The listing builds one solid part. Answer for the finished solid, in the listing's coordinates (mm). Face numbers are marked on the shaded views. Round coordinates to 2 decimals unless told otherwise and drop trailing zeros.
(1) A cutting plane is placed at A-A, the plane y = 14. Give the number of separate pieces and of enclosed holes in the cut face, and give its area (3 significant figures).
(2) Each of these flat-tipped pins is pushed along its axis until it touches: pin 1 Ø8 at (x, z) = (-48.01, -44.53) entering from +Y (3 decimals); pin 2 Ø3 at (x, z) = (-46, -40.5) entering from -Y (3 decimals); pin 3 Ø8.5 at (x, z) = (60.71, -57.23) entering from -Y. Where does it stop, or does it pass through?
(3) The mould has two halves that part along Z. Classify the marked faces 1, 2, 3 and 4: +Z half, -Z half, draft (parallel to the pull), parting line (faces both ways), or undercut.
(4) Find the intervals of material crossed by probe 1 along X at (y, z) = (12.5, -33.5); probe 2 along Z at (x, y) = (23, 18.5); probe 3 along Z at (x, y) = (-25.4, 12.5), in increasing order.
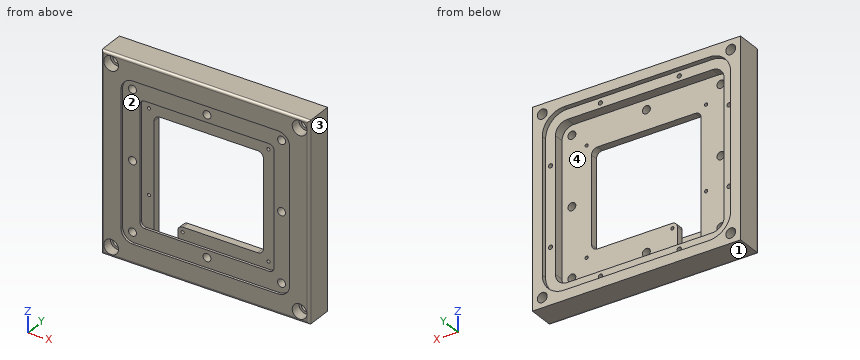
from build123d import *

# Parameters (mm, degrees)
SKETCH2_W                                            = 134.112
SKETCH2_H                                            = 127.1524
SKETCH2_W_2                                          = 83.312
SKETCH2_H_2                                          = 76.3524
SKETCH2_W_3                                          = 21.7424
SKETCH2_H_3                                          = 15.9766
BOSS_EXTRUDE1_DEPTH                                  = 15.875
BOSS_EXTRUDE2_DEPTH                                  = 9.525
CUT_EXTRUDE2_DEPTH                                   = 3.175
M2_5X0_45_TAPPED_HOLE1_D                             = 2.05
M2_5X0_45_TAPPED_HOLE1_DEPTH                         = 6.35
M2_5X0_45_TAPPED_HOLE1_TIP                           = 0.615882135
F_10_CLEARANCE_HOLE1_D                               = 5.1054
CUT_EXTRUDE3_DEPTH                                   = 6.35
CUT_EXTRUDE4_DEPTH                                   = 1.6
SKETCH12_W                                           = 70.612
SKETCH12_H                                           = 63.6524
CUT_EXTRUDE5_DEPTH                                   = 12.1
FILLET1_R                                            = 3.81
SKETCH13_W                                           = 134.112
SKETCH13_H                                           = 127.1524
CUT_EXTRUDE6_DEPTH                                   = 1.5875
FILLET2_R                                            = 1.5875
SKETCH14_W                                           = 15.3924
SKETCH14_H                                           = 22.86
CUT_EXTRUDE7_DEPTH                                   = 4.75
FILLET3_R                                            = 3.175
SKETCH15_W                                           = 134.112
SKETCH15_H                                           = 127.1524
BOSS_EXTRUDE3_DEPTH                                  = 3.175
F_6_32_TAPPED_HOLE1_AT_2_COUNT                       = 2
F_6_32_TAPPED_HOLE1_AT_2_PITCH                       = 108.1024
F_6_32_TAPPED_HOLE1_AT_3_COUNT                       = 2
F_6_32_TAPPED_HOLE1_AT_3_PITCH                       = 85.702359025
F_6_32_TAPPED_HOLE1_AT_4_COUNT                       = 2
F_6_32_TAPPED_HOLE1_AT_4_PITCH                       = 43.049882955
CBORE_FOR_1_4_BINDING_HEAD_MACHINE_SCREW_D           = 6.35
CBORE_FOR_1_4_BINDING_HEAD_MACHINE_SCREW_DEPTH       = 17.4625
CBORE_FOR_1_4_BINDING_HEAD_MACHINE_SCREW_CBORE_D     = 9.525
CBORE_FOR_1_4_BINDING_HEAD_MACHINE_SCREW_CBORE_DEPTH = 6.35


with BuildPart() as part:
    # Sketch2 → Boss-Extrude1 (new body)
    with BuildSketch(Plane(origin=(0, 0, 0), x_dir=(1, 0, 0), z_dir=(0, 1, 0))):
        Rectangle(SKETCH2_W, SKETCH2_H)
        Rectangle(SKETCH2_W_2, SKETCH2_H_2, mode=Mode.SUBTRACT)
        with Locations((-30.7848, 30.1879)):
            Rectangle(SKETCH2_W_3, SKETCH2_H_3)
    extrude(amount=BOSS_EXTRUDE1_DEPTH)

    # Sketch4 → Boss-Extrude2 (add)
    with BuildSketch(Plane(origin=(0, 0, 0), x_dir=(1, 0, 0), z_dir=(0, 1, 0))):
        Polygon((41.656, -38.1762), (41.656, 38.1762), (-19.9136, 38.1762), (-19.9136, 22.1996), (-41.656, 22.1996), (-41.656, -38.1762), align=None)
        Polygon((35.306, 31.8262), (-13.5636, 31.8262), (-13.5636, 15.8496), (-35.306, 15.8496), (-35.306, -31.8262), (35.306, -31.8262), align=None, mode=Mode.SUBTRACT)
    extrude(amount=BOSS_EXTRUDE2_DEPTH)

    # Sketch5 → Cut-Extrude2 (cut)
    with BuildSketch(Plane.XZ):
        with BuildLine():
            Line((46.736, -50.8762), (-46.736, -50.8762))
            ThreePointArc((-46.736, -50.8762), (-52.124153673, -48.644353673), (-54.356, -43.2562))
            Line((-54.356, -43.2562), (-54.356, 43.2562))
            ThreePointArc((-54.356, 43.2562), (-52.124153673, 48.644353673), (-46.736, 50.8762))
            Line((-46.736, 50.8762), (46.736, 50.8762))
            ThreePointArc((46.736, 50.8762), (52.124153673, 48.644353673), (54.356, 43.2562))
            Line((54.356, 43.2562), (54.356, -43.2562))
            ThreePointArc((54.356, -43.2562), (52.124153673, -48.644353673), (46.736, -50.8762))
        make_face()
    extrude(amount=-CUT_EXTRUDE2_DEPTH, mode=Mode.SUBTRACT)

    # M2.5x0.45 Tapped Hole1
    with Locations(Plane(origin=(0, 3.175, 0), x_dir=(-1, 0, 0), z_dir=(0, -1, 0))):
        with Locations((38.481, -35.0012), (-38.481, -35.0012), (38.481, 19.0246), (16.7386, 35.0012), (-38.481, 35.0012)):
            Hole(M2_5X0_45_TAPPED_HOLE1_D / 2, depth=M2_5X0_45_TAPPED_HOLE1_DEPTH)
            with Locations((0, 0, -(M2_5X0_45_TAPPED_HOLE1_DEPTH + M2_5X0_45_TAPPED_HOLE1_TIP / 2))):  # 118° drill point
                Cone(0, M2_5X0_45_TAPPED_HOLE1_D / 2, M2_5X0_45_TAPPED_HOLE1_TIP, mode=Mode.SUBTRACT)

    # 10 Clearance Hole1 (through all)
    with Locations(Plane(origin=(0, 3.175, 0), x_dir=(-1, 0, 0), z_dir=(0, -1, 0))):
        with Locations((48.006, -44.5262), (0, -44.5262), (-48.006, -44.5262), (-48.006, 0), (-48.006, 44.5262), (0, 44.5262), (48.006, 44.5262), (48.006, 0)):
            Hole(F_10_CLEARANCE_HOLE1_D / 2)

    # Sketch10 → Cut-Extrude3 (cut)
    with BuildSketch(Plane(origin=(0, 15.875, 0), x_dir=(1, 0, 0), z_dir=(0, 1, 0))):
        with BuildLine():
            Line((54.356, -43.2562), (54.356, 43.2562))
            ThreePointArc((54.356, 43.2562), (52.124153673, 48.644353673), (46.736, 50.8762))
            Line((46.736, 50.8762), (-46.736, 50.8762))
            ThreePointArc((-46.736, 50.8762), (-52.124153673, 48.644353673), (-54.356, 43.2562))
            Line((-54.356, 43.2562), (-54.356, -43.2562))
            ThreePointArc((-54.356, -43.2562), (-52.124153673, -48.644353673), (-46.736, -50.8762))
            Line((-46.736, -50.8762), (46.736, -50.8762))
            ThreePointArc((46.736, -50.8762), (52.124153673, -48.644353673), (54.356, -43.2562))
        make_face()
    extrude(amount=-CUT_EXTRUDE3_DEPTH, mode=Mode.SUBTRACT)

    # Sketch11 → Cut-Extrude4 (cut)
    with BuildSketch(Plane.XZ.offset(-3.175)):
        with BuildLine():
            Line((40.0685, 39.7637), (-40.0685, 39.7637))
            ThreePointArc((-40.0685, 39.7637), (-42.31356403, 38.83376403), (-43.2435, 36.5887))
            Line((-43.2435, 36.5887), (-43.2435, -36.5887))
            ThreePointArc((-43.2435, -36.5887), (-42.31356403, -38.83376403), (-40.0685, -39.7637))
            Line((-40.0685, -39.7637), (40.0685, -39.7637))
            ThreePointArc((40.0685, -39.7637), (42.31356403, -38.83376403), (43.2435, -36.5887))
            Line((43.2435, -36.5887), (43.2435, 36.5887))
            ThreePointArc((43.2435, 36.5887), (42.31356403, 38.83376403), (40.0685, 39.7637))
        make_face()
    extrude(amount=-CUT_EXTRUDE4_DEPTH, mode=Mode.SUBTRACT)

    # Sketch12 → Cut-Extrude5 (cut, through all)
    with BuildSketch(Plane.XZ.offset(-4.775)):
        Rectangle(SKETCH12_W, SKETCH12_H)
    extrude(amount=-CUT_EXTRUDE5_DEPTH, mode=Mode.SUBTRACT)

    # Fillet1
    fillet1_edges = [part.edges().sort_by_distance(p)[0] for p in [
        (-35.306, 7.15, -31.8262),
        (35.306, 7.15, -31.8262),
        (-35.306, 7.15, 31.8262),
        (35.306, 7.15, 31.8262),
    ]]
    fillet(fillet1_edges, radius=FILLET1_R)

    # Sketch13 → Cut-Extrude6 (cut)
    with BuildSketch(Plane.XZ):
        Rectangle(SKETCH13_W, SKETCH13_H)
        with BuildLine():
            Line((54.356, -43.2562), (54.356, 43.2562))
            ThreePointArc((54.356, 43.2562), (52.124153673, 48.644353673), (46.736, 50.8762))
            Line((46.736, 50.8762), (-46.736, 50.8762))
            ThreePointArc((-46.736, 50.8762), (-52.124153673, 48.644353673), (-54.356, 43.2562))
            Line((-54.356, 43.2562), (-54.356, -43.2562))
            ThreePointArc((-54.356, -43.2562), (-52.124153673, -48.644353673), (-46.736, -50.8762))
            Line((-46.736, -50.8762), (46.736, -50.8762))
            ThreePointArc((46.736, -50.8762), (52.124153673, -48.644353673), (54.356, -43.2562))
        make_face(mode=Mode.SUBTRACT)
    extrude(amount=-CUT_EXTRUDE6_DEPTH, mode=Mode.SUBTRACT)

    # Fillet2
    fillet2_edges = [part.edges().sort_by_distance(p)[0] for p in [
        (67.056, 1.5875, 0),
        (0, 1.5875, -63.5762),
        (-67.056, 1.5875, 0),
        (0, 1.5875, 63.5762),
    ]]
    fillet(fillet2_edges, radius=FILLET2_R)

    # Sketch14 → Cut-Extrude7 (cut)
    with BuildSketch(Plane(origin=(0, 9.525, 0), x_dir=(1, 0, 0), z_dir=(0, 1, 0))):
        with Locations((-27.6098, 39.4462)):
            Rectangle(SKETCH14_W, SKETCH14_H)
    extrude(amount=-CUT_EXTRUDE7_DEPTH, mode=Mode.SUBTRACT)

    # Fillet3
    fillet3_edges = [part.edges().sort_by_distance(p)[0] for p in [
        (-19.9136, 7.15, -31.8262),
        (-19.9136, 7.15, -50.8762),
        (-35.306, 7.15, -50.8762),
    ]]
    fillet(fillet3_edges, radius=FILLET3_R)

    # Sketch15 → Boss-Extrude3 (add)
    with BuildSketch(Plane(origin=(0, 15.875, 0), x_dir=(1, 0, 0), z_dir=(0, 1, 0))):
        Rectangle(SKETCH15_W, SKETCH15_H)
        with BuildLine():
            ThreePointArc((46.736, -57.2262), (56.614281733, -53.134481733), (60.706, -43.2562))
            Line((60.706, -43.2562), (60.706, 43.2562))
            ThreePointArc((60.706, 43.2562), (56.614281733, 53.134481733), (46.736, 57.2262))
            Line((46.736, 57.2262), (-46.736, 57.2262))
            ThreePointArc((-46.736, 57.2262), (-56.614281733, 53.134481733), (-60.706, 43.2562))
            Line((-60.706, 43.2562), (-60.706, -43.2562))
            ThreePointArc((-60.706, -43.2562), (-56.614281733, -53.134481733), (-46.736, -57.2262))
            Line((-46.736, -57.2262), (46.736, -57.2262))
        make_face(mode=Mode.SUBTRACT)
    extrude(amount=BOSS_EXTRUDE3_DEPTH)

    # Sketch18 → 6-32 Tapped Hole1 (revolve, cut)
    with BuildSketch(Plane(origin=(-25.4, 15.875, 54.0512), x_dir=(0, 0, 1), z_dir=(1, 0, 0))):
        Polygon((0, 0), (0, 10.33769403), (1.35255, 9.525), (1.35255, 0), align=None)
    f_6_32_tapped_hole1 = revolve(axis=Axis((-25.4, 22.225, 54.0512), (0, -1, 0)), mode=Mode.SUBTRACT)

    # 6-32 Tapped Hole1 at 2: 6-32 Tapped Hole1 ×2
    with Locations(*[(0, 0, -i * F_6_32_TAPPED_HOLE1_AT_2_PITCH) for i in range(1, F_6_32_TAPPED_HOLE1_AT_2_COUNT)]):
        add(f_6_32_tapped_hole1, mode=Mode.SUBTRACT)

    # 6-32 Tapped Hole1 at 3: 6-32 Tapped Hole1 ×2
    with Locations(*[Vector(-0.374913834, 0, -0.927059662) * (i * F_6_32_TAPPED_HOLE1_AT_3_PITCH) for i in range(1, F_6_32_TAPPED_HOLE1_AT_3_COUNT)]):
        add(f_6_32_tapped_hole1, mode=Mode.SUBTRACT)

    # 6-32 Tapped Hole1 at 4: 6-32 Tapped Hole1 ×2
    with Locations(*[Vector(-0.746366721, 0, -0.665534911) * (i * F_6_32_TAPPED_HOLE1_AT_4_PITCH) for i in range(1, F_6_32_TAPPED_HOLE1_AT_4_COUNT)]):
        add(f_6_32_tapped_hole1, mode=Mode.SUBTRACT)

    # Mirror1: 6-32 Tapped Hole1 across plane
    add(f_6_32_tapped_hole1.mirror(Plane(origin=(0, 0, 0), x_dir=(0, 0, 1), z_dir=(1, 0, 0))), mode=Mode.SUBTRACT)

    # Mirror1 copy 1 sketch → Mirror1 copy 1 (revolve, cut)
    with BuildSketch(Plane(origin=(25.4, 15.875, -54.0512), x_dir=(0, 0, 1), z_dir=(-1, 0, 0))):
        Polygon((0, 0), (0, -10.33769403), (1.35255, -9.525), (1.35255, 0), align=None)
    revolve(axis=Axis((25.4, 22.225, -54.0512), (0, 1, 0)), mode=Mode.SUBTRACT)

    # Mirror1 copy 2 sketch → Mirror1 copy 2 (revolve, cut)
    with BuildSketch(Plane(origin=(57.531, 15.875, -25.4), x_dir=(0, 0, 1), z_dir=(-1, 0, 0))):
        Polygon((0, 0), (0, -10.33769403), (1.35255, -9.525), (1.35255, 0), align=None)
    revolve(axis=Axis((57.531, 22.225, -25.4), (0, 1, 0)), mode=Mode.SUBTRACT)

    # Mirror1 copy 3 sketch → Mirror1 copy 3 (revolve, cut)
    with BuildSketch(Plane(origin=(57.531, 15.875, 25.4), x_dir=(0, 0, 1), z_dir=(-1, 0, 0))):
        Polygon((0, 0), (0, -10.33769403), (1.35255, -9.525), (1.35255, 0), align=None)
    revolve(axis=Axis((57.531, 22.225, 25.4), (0, 1, 0)), mode=Mode.SUBTRACT)

    # CBORE for 1_4 Binding Head Machine Screw
    with Locations(Plane(origin=(0, 1.5875, 0), x_dir=(-1, 0, 0), z_dir=(0, -1, 0))):
        with Locations((60.706, -57.2262), (-60.706, -57.2262), (-60.706, 57.2262), (60.706, 57.2262)):
            CounterBoreHole(CBORE_FOR_1_4_BINDING_HEAD_MACHINE_SCREW_D / 2, CBORE_FOR_1_4_BINDING_HEAD_MACHINE_SCREW_CBORE_D / 2, CBORE_FOR_1_4_BINDING_HEAD_MACHINE_SCREW_CBORE_DEPTH, depth=CBORE_FOR_1_4_BINDING_HEAD_MACHINE_SCREW_DEPTH)


solid = part.part
Solutions:
1. separate pieces: 1
1. enclosed holes: 13
1. area: 5,870 mm2
2. pin 1: stops at y = 9.525
2. pin 2: stops at y = 3.175
2. pin 3: stops at y = 7.94
3. face 1: -Z half
3. face 2: undercut
3. face 3: draft
3. face 4: undercut
4. probe 1: x = -67.06 to -54.36, 54.36 to 67.06
4. probe 2: z = -63.58 to -57.23, 57.23 to 63.58
4. probe 3: z = -63.58 to -55.4, -52.7 to -50.88, 50.88 to 52.7, 55.4 to 63.58
